```python
from build123d import *

# Parameters (mm, degrees)
ESBO_O1_W                = 6.74
ESBO_O1_H                = 8
ESBO_O1_W_2              = 6.65
RESSALTO_EXTRUS_O1_DEPTH = 10


with BuildPart() as part:
    # Esboço1 → Ressalto-extrusão1 (new body)
    # profile 1 of 3: a face of its own
    with BuildSketch(Plane(origin=(0, 0, 0), x_dir=(1, 0, 0), z_dir=(0, 1, 0))):
        with BuildLine():
            Line((18.75, 5.2), (-18.75, 5.2))
            ThreePointArc((-18.75, 5.2), (-20.164213562, 4.614213562), (-20.75, 3.2))
            Line((-20.75, 3.2), (-20.75, 0.7))
            Line((-20.75, 0.7), (-20.75, -1.3))
            Line((-20.75, -1.3), (-20.75, -3.2))
            ThreePointArc((-20.75, -3.2), (-20.164213562, -4.614213562), (-18.75, -5.2))
            Line((-18.75, -5.2), (18.75, -5.2))
            ThreePointArc((18.75, -5.2), (20.164213562, -4.614213562), (20.75, -3.2))
            Line((20.75, -3.2), (20.75, -1.3))
            Line((20.75, -1.3), (20.75, 0.7))
            Line((20.75, 0.7), (20.75, 3.2))
            ThreePointArc((20.75, 3.2), (20.164213562, 4.614213562), (18.75, 5.2))
        make_face()
        with Locations((-15.88, 0)):
            Rectangle(ESBO_O1_W, ESBO_O1_H, mode=Mode.SUBTRACT)
        with Locations((-7.94, 0)):
            Rectangle(ESBO_O1_W, ESBO_O1_H, mode=Mode.SUBTRACT)
        Rectangle(ESBO_O1_W, ESBO_O1_H, mode=Mode.SUBTRACT)
        with Locations((7.94, 0)):
            Rectangle(ESBO_O1_W, ESBO_O1_H, mode=Mode.SUBTRACT)
        with Locations((15.88, 0)):
            Rectangle(ESBO_O1_W, ESBO_O1_H, mode=Mode.SUBTRACT)
    # profile 2 of 3: a face of its own
    with BuildSketch(Plane(origin=(0, 0, 0), x_dir=(1, 0, 0), z_dir=(0, 1, 0))):
        with BuildLine():
            Line((-20.75, -1.3), (-20.75, 0.7))
            Line((-20.75, 0.7), (-31.75, 0.7))
            ThreePointArc((-31.75, 0.7), (-33.164213562, 0.114213562), (-33.75, -1.3))
            Line((-33.75, -1.3), (-33.75, -14.642724204))
            Line((-33.75, -14.642724204), (-33.75, -16))
            Line((-33.75, -16), (-33.75, -16.3))
            Line((-33.75, -16.3), (-33.75, -17.5))
            Line((-33.75, -17.5), (-33.75, -25.5))
            Line((-33.75, -25.5), (-33.75, -26.7))
            Line((-33.75, -26.7), (-17.75, -26.7))
            ThreePointArc((-17.75, -26.7), (-16.335786438, -26.114213562), (-15.75, -24.7))
            Line((-15.75, -24.7), (-15.75, -18.3))
            ThreePointArc((-15.75, -18.3), (-16.335786438, -16.885786438), (-17.75, -16.3))
            Line((-17.75, -16.3), (-31.75, -16.3))
            Line((-31.75, -16.3), (-31.75, -16))
            Line((-31.75, -16), (-31.75, -3.3))
            ThreePointArc((-31.75, -3.3), (-31.164213562, -1.885786438), (-29.75, -1.3))
            Line((-29.75, -1.3), (-20.75, -1.3))
        make_face()
        with Locations((-28.425, -21.5)):
            Rectangle(ESBO_O1_W_2, ESBO_O1_H, mode=Mode.SUBTRACT)
        with Locations((-20.575, -21.5)):
            Rectangle(ESBO_O1_W_2, ESBO_O1_H, mode=Mode.SUBTRACT)
    # profile 3 of 3: a face of its own
    with BuildSketch(Plane(origin=(0, 0, 0), x_dir=(1, 0, 0), z_dir=(0, 1, 0))):
        with BuildLine():
            Line((31.75, 0.7), (20.75, 0.7))
            Line((20.75, 0.7), (20.75, -1.3))
            Line((20.75, -1.3), (29.75, -1.3))
            ThreePointArc((29.75, -1.3), (31.164213562, -1.885786438), (31.75, -3.3))
            Line((31.75, -3.3), (31.75, -16))
            Line((31.75, -16), (31.75, -16.3))
            Line((31.75, -16.3), (17.75, -16.3))
            ThreePointArc((17.75, -16.3), (16.335786438, -16.885786438), (15.75, -18.3))
            Line((15.75, -18.3), (15.75, -24.7))
            ThreePointArc((15.75, -24.7), (16.335786438, -26.114213562), (17.75, -26.7))
            Line((17.75, -26.7), (33.75, -26.7))
            Line((33.75, -26.7), (33.75, -25.5))
            Line((33.75, -25.5), (33.75, -17.5))
            Line((33.75, -17.5), (33.75, -16.3))
            Line((33.75, -16.3), (33.75, -16))
            Line((33.75, -16), (33.75, -14.642724204))
            Line((33.75, -14.642724204), (33.75, -1.3))
            ThreePointArc((33.75, -1.3), (33.164213562, 0.114213562), (31.75, 0.7))
        make_face()
        with Locations((20.575, -21.5)):
            Rectangle(ESBO_O1_W_2, ESBO_O1_H, mode=Mode.SUBTRACT)
        with Locations((28.425, -21.5)):
            Rectangle(ESBO_O1_W_2, ESBO_O1_H, mode=Mode.SUBTRACT)
    extrude(amount=RESSALTO_EXTRUS_O1_DEPTH)


solid = part.part
```
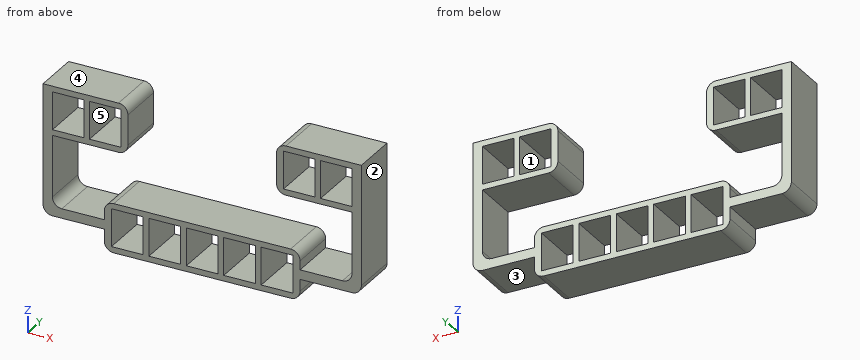
Geometry check sheet. Reference: the model listing, model coordinates, mm. Face numbers are marked on the shaded views. A direction names the side the tool comes from. Round coordinates to 2 decimals unless told otherwise and drop trailing zeros. Write each loop counter-clockwise with the first axis right and the second up, starting at its lowest first coordinate (ties: lowest second). Pieces come first, ordered by that corner, then holes. Notation, with made-up numbers: (26.25, 18.5) - (78.25, 18.5) arc R21 cw to (78.25, 53.5) - close; hole circle Ø9 at (60, 29.5). An arc over 180 degrees is marked (long way). Write each question's results on one line, items separated by ' | '.
(1) Sectioned sample at A-A, the plane z = 8. Enter the section's corners in (x, y).
Computed:
outline: (-33.75, 0) - (-31.75, 0) - (-31.75, 10) - (-33.75, 10) - close; (31.75, 0) - (33.75, 0) - (33.75, 10) - (31.75, 10) - close
(2) Thickness scan on probe 1 along Z at (x, y) = (-19, 9.5); probe 2 along Z at (x, y) = (30, 4); probe 3 along X at (y, z) = (3.5, 23). Record the ranges inside material, lowest first. Write a range as from..to.
Computed:
probe 1: z = -5.18..-4, 4..5.18, 16.3..17.5, 25.5..26.7 | probe 2: z = -0.7..1.32, 16.3..17.5, 25.5..26.7 | probe 3: x = -33.75..-31.75, -25.1..-23.9, -17.25..-15.75, 15.75..17.25, 23.9..25.1, 31.75..33.75
(3) Sectioned sample at B-B, the plane x = 28.5. Enter the section's corners in (y, z), plus the area to 3 significant figures.
Computed:
outline: (0, -0.7) - (10, -0.7) - (10, 1.3) - (0, 1.3) - close; (0, 16.3) - (10, 16.3) - (10, 17.5) - (0, 17.5) - close; (0, 25.5) - (10, 25.5) - (10, 26.7) - (0, 26.7) - close | area: 44.0 mm^2
(4) Depth check by flat-ended pin: pin 1 Ø4 at (y, z) = (5, -2) entering from -X; pin 2 Ø8 at (x, z) = (-12.5, 10.5) entering from +Y; pin 3 Ø3.5 at (x, y) = (-7, 7) entering from +Z; pin 4 Ø4 at (x, y) = (-23, 7) entering from -Z. Enter the tip coordinate at first touch or a pass-through.
Computed:
pin 1: stops at x = -33.27 | pin 2: passes through | pin 3: stops at z = 5.2 | pin 4: stops at z = -0.7
(5) Draft check along X on the marked faces 1, 2 and 3. Enter one of: pulls with the +X half, pulls with the -X half, needs draft (parallel to the pull), parting line crosses it, or undercut.
Computed:
face 1: undercut | face 2: pulls with the +X half | face 3: needs draft
(6) Sectioned sample at C-C, the plane y = 5. Count the separate pieces of the cut face and the enclosed holes in it, plus the area to 3 significant figures.
Computed:
separate pieces: 1 | enclosed holes: 9 | area: 429 mm^2
(7) Set-up check for the marked faces 4 and 5: record each of +Z, -Z, +X, -X, +Y, -Y from which the full face is reachable in a straight line by a thin tool's end or side.
Computed:
face 4: +Z, +X, -X, +Y, -Y | face 5: +Y, -Y
